Could you check a few things on this model? Use its own coordinates, in mm. Round coordinates to 2 decimals unless told otherwise and drop trailing zeros. Write each loop counter-clockwise with the first axis right and the second up, starting at its lowest first coordinate (ties: lowest second). Pieces come first, ordered by that corner, then holes. Notation, with made-up numbers: M 8,73 L 38,73 A18 ccw 38,81 Z; hole C 60,4.25 d11. An arc over 180 degrees is marked long. One line per item, written item: value. Start each with the question number.
(1) I want a section at C-C on x = 17. Please give me the cut outline in (y, z).
(2) I want a section at B-B on z = -12. Please give me the cut outline in (x, y), and give its area (3 significant figures).
(3) I want a section at A-A on y = 2.5. Please give me the cut outline in (x, z).
(4) I want a section at D-D on y = 14. Please give me the cut outline in (x, z), and give its area (3 significant figures).
(5) If I drill on L1, parallel to Z at x = 52, y = 3.5; L2, parallel to Y at x = 56.5, z = -17.5; L3, parallel to X at y = 12.75, z = -1, over which ranges is the centre line in solid material (lowest first)?
(6) I'm going to push flat-ended pins straight in: pin 1 Ø6 at (y, z) = (13, -23.5) entering from +X; pin 2 Ø3 at (y, z) = (13.5, -59.5) entering from +X. Where does each tip first touch, or does it pass through?
```python
from build123d import *

# Parameters (mm, degrees)
SKETCH_1_W      = 50
SKETCH_1_H      = 16
EXTRUDE_1_DEPTH = 95
FILLET_1_R      = 2
SKETCH_2_R      = 4
EXTRUDE_2_DEPTH = 5


with BuildPart() as part:
    # 草图1 → 凸台-拉伸1 (new body)
    with BuildSketch(Plane.XY):
        with Locations((25, 8)):
            Rectangle(SKETCH_1_W, SKETCH_1_H)
        Polygon((62, 0), (62, 6), (50, 16), (50, 0), align=None)
    extrude(amount=-EXTRUDE_1_DEPTH)

    # 圆角1
    fillet_1_edges = [part.edges().sort_by_distance(p)[0] for p in [
        (62, 3, -95),
        (0, 8, -95),
        (0, 8, 0),
        (62, 3, 0),
    ]]
    fillet(fillet_1_edges, radius=FILLET_1_R)

    # 草图2 → 凸台-拉伸2 (add)
    with BuildSketch(Plane.XY):
        with Locations((17, 8)):
            Circle(SKETCH_2_R)
        with Locations((34, 8)):
            Circle(SKETCH_2_R)
    extrude(amount=EXTRUDE_2_DEPTH)


solid = part.part
```
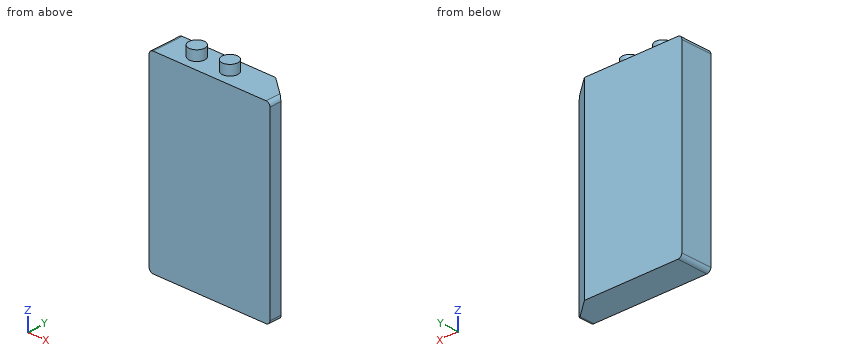
Found:
1. outline: M 0,-95 L 16,-95 L 16,0 L 12,0 L 12,5 L 4,5 L 4,0 L 0,0 Z
2. outline: M 0,0 L 62,0 L 62,6 L 50,16 L 0,16 Z
2. area: 932 mm²
3. outline: M 0,-93 A2 ccw 2,-95 L 60,-95 A2 ccw 62,-93 L 62,-2 A2 ccw 60,0 L 2,0 A2 ccw 0,-2 Z
4. outline: M 0,-93 A2 ccw 2,-95 L 52.4,-95 L 52.4,0 L 2,0 A2 ccw 0,-2 Z
4. area: 4,980 mm²
5. L1: z = -95 to 0
5. L2: y = 0 to 10.58
5. L3: x = 0.27 to 53.9
6. pin 1: stops at x = 57.2
6. pin 2: stops at x = 54.8
